CAD build for the part. Positions are in the model's coordinates, mm. Face numbers are marked on the shaded views. A direction names the side the tool comes from. Give positions to 0.01 mm unless a question says otherwise; leave off trailing zeros. Loops run counter-clockwise (first coordinate to the right, second up) from the corner with the lowest first, then second, coordinate; pieces in that order, holes last. Notation, with made-up numbers: (8.25, 79) - (14.25, 79) arc R19 ccw to (14.25, 85) - close; hole circle Ø10 at (20.25, 14). An arc over 180 degrees is marked (long way). Return JSON: item names as keys, results as strings.
from build123d import *

# Parameters (mm, degrees)
CROQUIS1_R              = 7
SALIENTE_EXTRUIR1_DEPTH = 2
CROQUIS2_R              = 5
SALIENTE_EXTRUIR2_DEPTH = 8
CROQUIS3_R              = 2.5
CORTAR_EXTRUIR1_DEPTH   = 18
REDONDEO1_R             = 0.25


with BuildPart() as part:
    # Croquis1 → Saliente-Extruir1 (new body)
    with BuildSketch(Plane(origin=(0, 0, 0), x_dir=(1, 0, 0), z_dir=(0, 1, 0))):
        Circle(CROQUIS1_R)
    extrude(amount=SALIENTE_EXTRUIR1_DEPTH)

    # Croquis2 → Saliente-Extruir2 (add)
    with BuildSketch(Plane(origin=(0, 2, 0), x_dir=(1, 0, 0), z_dir=(0, 1, 0))):
        Circle(CROQUIS2_R)
    extrude(amount=SALIENTE_EXTRUIR2_DEPTH)

    # Croquis3 → Cortar-Extruir1 (cut)
    with BuildSketch(Plane(origin=(0, 10, 0), x_dir=(1, 0, 0), z_dir=(0, 1, 0))):
        Circle(CROQUIS3_R)
    extrude(amount=-CORTAR_EXTRUIR1_DEPTH, mode=Mode.SUBTRACT)

    # Redondeo1
    redondeo1_edges = [part.edges().sort_by_distance(p)[0] for p in [
        (-7, 0, 0),
        (-7, 2, 0),
        (-5, 2, 0),
        (-5, 10, 0),
    ]]
    fillet(redondeo1_edges, radius=REDONDEO1_R)


solid = part.part
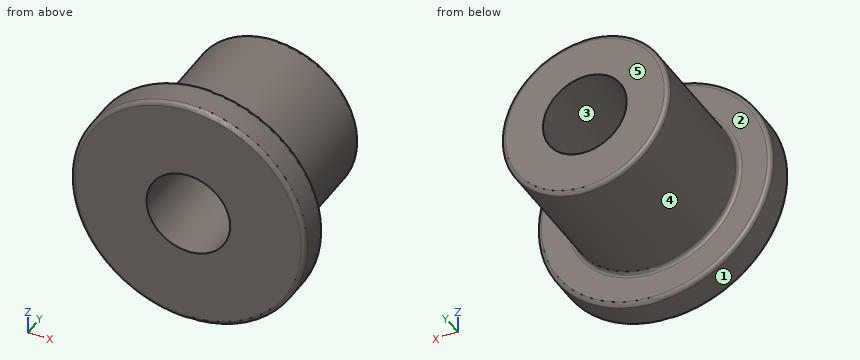
1. Pull direction Z, two halves, no side cores. Call the marked faces 3, 4 and 5: +Z half, -Z half, draft (parallel to the pull), parting line (faces both ways), or undercut.
Values follow:
{"face 3": "undercut", "face 4": "parting line", "face 5": "draft"}
2. Cut at C-C, the plane y = 3.25. Write the cut outline in (x, z).
Values follow:
{"outline": "circle Ø10 at (0, 0); hole circle Ø5 at (0, 0)"}
3. Cut at B-B, the plane x = 0. Write the cut outline in (y, z).
Values follow:
{"outline": "(0, -6.75) arc R0.25 ccw to (0.25, -7) - (1.75, -7) arc R0.25 ccw to (2, -6.75) - (2, -5.25) arc R0.25 cw to (2.25, -5) - (9.75, -5) arc R0.25 ccw to (10, -4.75) - (10, -2.5) - (0, -2.5) - close; (0, 2.5) - (10, 2.5) - (10, 4.75) arc R0.25 ccw to (9.75, 5) - (2.25, 5) arc R0.25 cw to (2, 5.25) - (2, 6.75) arc R0.25 ccw to (1.75, 7) - (0.25, 7) arc R0.25 ccw to (0, 6.75) - close"}
4. Cut at A-A, the plane z = 0. Write the cut outline in (x, y), plus the area to 3 significant figures.
Values follow:
{"outline": "(-7, 0.25) arc R0.25 ccw to (-6.75, 0) - (-2.5, 0) - (-2.5, 10) - (-4.75, 10) arc R0.25 ccw to (-5, 9.75) - (-5, 2.25) arc R0.25 cw to (-5.25, 2) - (-6.75, 2) arc R0.25 ccw to (-7, 1.75) - close; (2.5, 0) - (6.75, 0) arc R0.25 ccw to (7, 0.25) - (7, 1.75) arc R0.25 ccw to (6.75, 2) - (5.25, 2) arc R0.25 cw to (5, 2.25) - (5, 9.75) arc R0.25 ccw to (4.75, 10) - (2.5, 10) - close", "area": "57.9 mm²"}
5. Drop flat-ended pins along their axis: P1, Ø3, axis at y = 4, z = 1.5, coming from the +X side; P2, Ø3, axis at y = 2.5, z = 2, coming from the -X side; P3, Ø3, axis at x = 4, y = 5, coming from the +Z side. Give the stop position or say it passes through.
Values follow:
{"P1": "stops at x = 5", "P2": "stops at x = -6.97", "P3": "stops at z = 4.33"}
6. Drill centre lines: probe 1 along X at (y, z) = (5, 0); probe 2 along X at (y, z) = (1, 0). Where is each one in solid material? Low to high.
Values follow:
{"probe 1": "x = -5 to -2.5, 2.5 to 5", "probe 2": "x = -7 to -2.5, 2.5 to 7"}
7. Which spindle directions (+Z, -Z, +X, -X, +Y, -Y) get a long thin tool onto all of the face, cutting with end or side? Do the marked faces 1 and 2. Say none if no direction does.
Values follow:
{"face 1": "+Y, -Y", "face 2": "+Y"}
